The listing builds one solid part. Answer for the finished solid, in the listing's coordinates (mm). A direction names the side the tool comes from. Coordinates: 2 decimals unless noted, no trailing zeros. Order: outer loops, then holes, each group sorted by start corner. A loop starts at its lowest first (then second) coordinate and runs counter-clockwise, first axis right, second up. Notation, with made-up numbers: (12.25, -20.75) -> (56.25, -20.75) arc R28 ccw to (56.25, 11.25) -> close; hole circle Ø6 at (-25, 88.25). An arc over 180 degrees is marked (long way). Write each question's results on one line, items separated by ' | '. Start each with the question number.
(1) The part is cut by section A-A, the plane y = 0. Count the separate pieces of the cut face and the enclosed holes in it, then the cut area to 3 significant figures.
(2) Given pin 1 (7 mm diameter, centred on y = 0, z = 35.5, fed in from -X); pin 2 (2 mm diameter, centred on x = 111.5, y = 8, fed in from +Z); pin 3 (5 mm diameter, centred on x = 103.5, z = -14, fed in from +Y); pin 4 (13.5 mm diameter, centred on y = -35.5, z = 0, fed in from +X), each flat-ended and moving along its own axis, determine where each tip first touches the part or whether it passes through.
(3) The part is cut by section C-C, the plane x = 18. Give the vertices of the cut face in (y, z).
(4) A tool of negligible diameter and unlimited length cuts with its end or side. For faces 1 (the face through (11.874, 0.187, 31.254)), 2 (the face through (105.37, 24.397, 12.69)), 3 (the face through (3, 27, 9)), from which of +Z, -Z, +X, -X, +Y, -Y can it reach the whole face along a straight path? Write none if from no direction.
(5) Straight lines are drawn through the part: L1, parallel to Y at x = 10, z = 0; L2, parallel to X at y = 22.5, z = -19; L3, parallel to Y at x = 14.5, z = -3. For each, find the intervals that lie inside material, in ascending order.
(6) The part is cut by section D-D, the plane x = 174.5. Give the vertices of the cut face in (y, z), then the cut area to 3 significant figures.
(7) Determine the mould class of faces 4 (the face through (11.874, 39.714, -0.553)), 5 (the face through (3.146, -12.659, 40.199)), 6 (the face through (11.874, -31.286, -0.553)), 7 (the face through (189, 0, 0)) for opening direction Z: +Z half, -Z half, draft (parallel to the pull), parting line (faces both ways), or undercut.
```python
from build123d import *

# Parameters (mm, degrees)
CHAMFER1_SIZE      = 3
CUT_EXTRUDE1_REACH = 198.586
SKETCH2_R          = 4.25


with BuildPart() as part:
    # Sketch1 → Revolve1 (revolve)
    with BuildSketch(Plane.XY, mode=Mode.PRIVATE) as revolve1_sk:
        Polygon((189, 0), (189, 20), (151, 20), (151, 27.5), (61, 27.5), (61, 30), (21, 30), (21, 45), (3, 45), (3, 28), (0, 25), (0, 0), align=None)
    revolve(revolve1_sk.sketch.rotate(Axis((0, 0, 0), (1, 0, 0)), 90), axis=Axis((0, 0, 0), (1, 0, 0)))

    # Chamfer1
    chamfer1_edges = [part.edges().sort_by_distance(p)[0] for p in [
        (3, 0, -45),
    ]]
    chamfer(chamfer1_edges, length=CHAMFER1_SIZE)

    # Sketch2 → Cut-Extrude1 (cut, up to next)
    with BuildSketch(Plane.ZY.offset(-3), mode=Mode.PRIVATE) as cut_extrude1_sk1:
        with Locations((35.5, 0)):
            Circle(SKETCH2_R)
    cut_extrude1_tool1 = extrude(cut_extrude1_sk1.sketch, amount=-CUT_EXTRUDE1_REACH, mode=Mode.PRIVATE) & part.part
    # Sketch2 → Cut-Extrude1 (cut, up to next)
    with BuildSketch(Plane.ZY.offset(-3), mode=Mode.PRIVATE) as cut_extrude1_sk2:
        with Locations((0, -35.5)):
            Circle(SKETCH2_R)
    cut_extrude1_tool2 = extrude(cut_extrude1_sk2.sketch, amount=-CUT_EXTRUDE1_REACH, mode=Mode.PRIVATE) & part.part
    # Sketch2 → Cut-Extrude1 (cut, up to next)
    with BuildSketch(Plane.ZY.offset(-3), mode=Mode.PRIVATE) as cut_extrude1_sk3:
        with Locations((-35.5, 0)):
            Circle(SKETCH2_R)
    cut_extrude1_tool3 = extrude(cut_extrude1_sk3.sketch, amount=-CUT_EXTRUDE1_REACH, mode=Mode.PRIVATE) & part.part
    # Sketch2 → Cut-Extrude1 (cut, up to next)
    with BuildSketch(Plane.ZY.offset(-3), mode=Mode.PRIVATE) as cut_extrude1_sk4:
        with Locations((0, 35.5)):
            Circle(SKETCH2_R)
    cut_extrude1_tool4 = extrude(cut_extrude1_sk4.sketch, amount=-CUT_EXTRUDE1_REACH, mode=Mode.PRIVATE) & part.part
    add(cut_extrude1_tool1.solids().sort_by_distance((3, 0, 35.5))[0], mode=Mode.SUBTRACT)
    add(cut_extrude1_tool2.solids().sort_by_distance((3, -35.5, 0))[0], mode=Mode.SUBTRACT)
    add(cut_extrude1_tool3.solids().sort_by_distance((3, 0, -35.5))[0], mode=Mode.SUBTRACT)
    add(cut_extrude1_tool4.solids().sort_by_distance((3, 35.5, 0))[0], mode=Mode.SUBTRACT)


solid = part.part
```
Established:
1) separate pieces: 3 | enclosed holes: 0 | area: 10,300 mm^2
2) pin 1: passes through | pin 2: stops at z = 26.59 | pin 3: stops at y = 24.98 | pin 4: stops at x = 61
3) outline: circle Ø90 at (0, 0); hole circle Ø8.5 at (-35.5, 0); hole circle Ø8.5 at (0, -35.5); hole circle Ø8.5 at (0, 35.5); hole circle Ø8.5 at (35.5, 0)
4) face 1: +X, -X | face 2: +X | face 3: -X
5) L1: y = -45 to -39.75, -31.25 to 31.25, 39.75 to 45 | L2: x = 3 to 61 | L3: y = -44.9 to -38.51, -32.49 to 32.49, 38.51 to 44.9
6) outline: circle Ø40 at (0, 0) | area: 1,260 mm^2
7) face 4: undercut | face 5: parting line | face 6: undercut | face 7: draft
